```python
from build123d import *

# Parameters (mm, degrees)
SKETCH1_R           = 14
SKETCH1_R_2         = 9
BOSS_EXTRUDE1_DEPTH = 35
SKETCH2_R           = 7.5
SKETCH2_R_2         = 4.5
BOSS_EXTRUDE2_DEPTH = 9.5
BOSS_EXTRUDE4_DEPTH = 2.5
RIB6_START          = -5
RIB6_DEPTH          = 10


with BuildPart() as part:
    # Sketch1 → Boss-Extrude1 (new body)
    with BuildSketch(Plane.XY):
        Circle(SKETCH1_R)
        Circle(SKETCH1_R_2, mode=Mode.SUBTRACT)
    extrude(amount=-BOSS_EXTRUDE1_DEPTH)



with BuildPart() as body_2:
    # Sketch2 → Boss-Extrude2 (new, symmetric)
    with BuildSketch(Plane(origin=(0, 0, 0), x_dir=(0, 0, -1), z_dir=(1, 0, 0))):
        with Locations((17.5, 26)):
            Circle(SKETCH2_R)
        with Locations((17.5, 26)):
            Circle(SKETCH2_R_2, mode=Mode.SUBTRACT)
    extrude(amount=BOSS_EXTRUDE2_DEPTH, both=True)


with BuildPart() as part_1:
    add(part.part)

    add(body_2.part)  # Boss-Extrude4 merges body 2
    # Sketch4 → Boss-Extrude4 (add, symmetric)
    with BuildSketch(Plane(origin=(0, 0, 0), x_dir=(0, 0, -1), z_dir=(1, 0, 0))):
        with BuildLine():
            Line((11.342086503, 30.281366763), (0, 13.967981008))
            Line((0, 13.967981008), (0, 13.516905435))
            Line((0, 13.516905435), (35, 13.771632184))
            Line((35, 13.771632184), (35, 13.967981008))
            Line((35, 13.967981008), (23.657913497, 30.281366763))
            ThreePointArc((23.657913497, 30.281366763), (24.65661761, 28.243395726), (25, 26))
            ThreePointArc((25, 26), (15.256604274, 18.84338239), (11.342086503, 30.281366763))
        make_face()
    extrude(amount=BOSS_EXTRUDE4_DEPTH, both=True)

    # Rib6: read off the stored shape, not the designer's step
    # Rib6 outline → Rib6 (add)
    with BuildSketch(Plane.XY.offset(-17.5).offset(RIB6_START)):
        with BuildLine():
            Line((9.5, 20.409830056), (2.5, 20.409830056))
            Line((2.5, 20.409830056), (2.5, 13.774977314))
            ThreePointArc((2.5, 13.774977314), (7.971087724, 11.509203296), (12.016061116, 7.18430757))
            Line((12.016061116, 7.18430757), (9.5, 18.509693936))
            Line((9.5, 18.509693936), (9.5, 20.409830056))
        make_face()
    extrude(amount=RIB6_DEPTH)


solid = part_1.part
```
Here's how the part is built. I have some questions about the finished solid (model axes, mm). A direction names the side the tool comes from. Coordinates: 2 decimals unless noted, no trailing zeros. Loops run counter-clockwise (first coordinate to the right, second up) from the corner with the lowest first, then second, coordinate; pieces in that order, holes last. Notation, with made-up numbers: (88, 53.5) -> (114, 53.5) arc R18 cw to (114, 79.5) -> close; hole circle Ø9 at (-5, 4). An arc over 180 degrees is marked (long way). Return JSON: item names as keys, results as strings.
1) Will these pins go through, and if not, where does the flat tip stop? pin 1 (8 mm diameter, centred on x = 1.5, y = 18.5, fed in from +Z); pin 2 (4.5 mm diameter, centred on y = 29.5, z = -14.5, fed in from +X); pin 3 (4.5 mm diameter, centred on y = 24.5, z = -19.5, fed in from -X).
Results below:
{"pin 1": "z = -0.37", "pin 2": "x = 9.5", "pin 3": "x = -9.5"}
2) If we section it at C-C, the plane y = 0: Write out the boundary of the cut face in (x, z), then the cut area to 3 significant figures.
Results below:
{"outline": "(-14, -35) -> (-9, -35) -> (-9, 0) -> (-14, 0) -> close; (9, -35) -> (14, -35) -> (14, 0) -> (9, 0) -> close", "area": "350 mm²"}
3) If we section it at D-D, the plane x = -6.5: Write out the boundary of the cut face in (y, z).
Results below:
{"outline": "(-12.4, -35) -> (-6.22, -35) -> (-6.22, 0) -> (-12.4, 0) -> close; (6.22, -35) -> (12.4, -35) -> (12.4, 0) -> (6.22, 0) -> close; circle Ø15 at (26, -17.5); hole circle Ø9 at (26, -17.5)"}
4) For faces 1 (the face through (2.5, 18, -8)), 2 (the face through (7, 15, -22.5)), 3 (the face through (-9.5, 26.1, -22.4)), 4 (the face through (-9, 3, -35)), which set-ups out of +Z, -Z, +X, -X, +Y, -Y let a thin tool reach every point of the face, with its end or its side?
Results below:
{"face 1": "+Z, +X", "face 2": "-Z, +X", "face 3": "+Z, -Z, -X, +Y", "face 4": "-Z, +X, -X, +Y, -Y"}
5) If we section it at A-A, the plane x = 0: Count the separate pieces of the cut face and the enclosed holes in it, then the cut area to 3 significant figures.
Results below:
{"separate pieces": "2", "enclosed holes": "1", "area": "699 mm²"}
6) I need wall thicknesses on line 1 (Y direction, x = 6, z = -11); line 2 (Y direction, x = -2, z = -17.5); line 3 (Y direction, x = 1.25, z = -11.5). Which ranges of each line are inside material? Lowest first, please. Write a range as from..to.
Results below:
{"line 1": "-12.65..-6.71, 6.71..12.65, 22.26..29.74", "line 2": "-13.86..-8.77, 8.77..21.5, 30.5..33.5", "line 3": "-13.94..-8.91, 8.91..30.5"}
7) If we section it at B-B, the plane z = -17.5: Write out the boundary of the cut face in (x, y).
Results below:
{"outline": "(-9.5, 18.5) -> (-2.5, 18.5) -> (-2.5, 13.77) arc R14 ccw (long way) to (12.02, 7.18) -> (9.5, 18.51) -> (9.5, 21.5) -> (-9.5, 21.5) -> close; (-9.5, 30.5) -> (9.5, 30.5) -> (9.5, 33.5) -> (-9.5, 33.5) -> close; hole circle Ø18 at (0, 0)"}
8) Thinking about a two-plate mould opening in X: for faces 5 (the face through (-1.172, 8.923, -17.255)), 6 (the face through (9.5, 21, -17)), 7 (the face through (-0.13, 29.04, -14.18)), 8 (the face through (-2.5, 18, -17)), which applies, +X half, -X half, draft (parallel to the pull), parting line (faces both ways), or undercut?
Results below:
{"face 5": "undercut", "face 6": "+X half", "face 7": "draft", "face 8": "-X half"}
